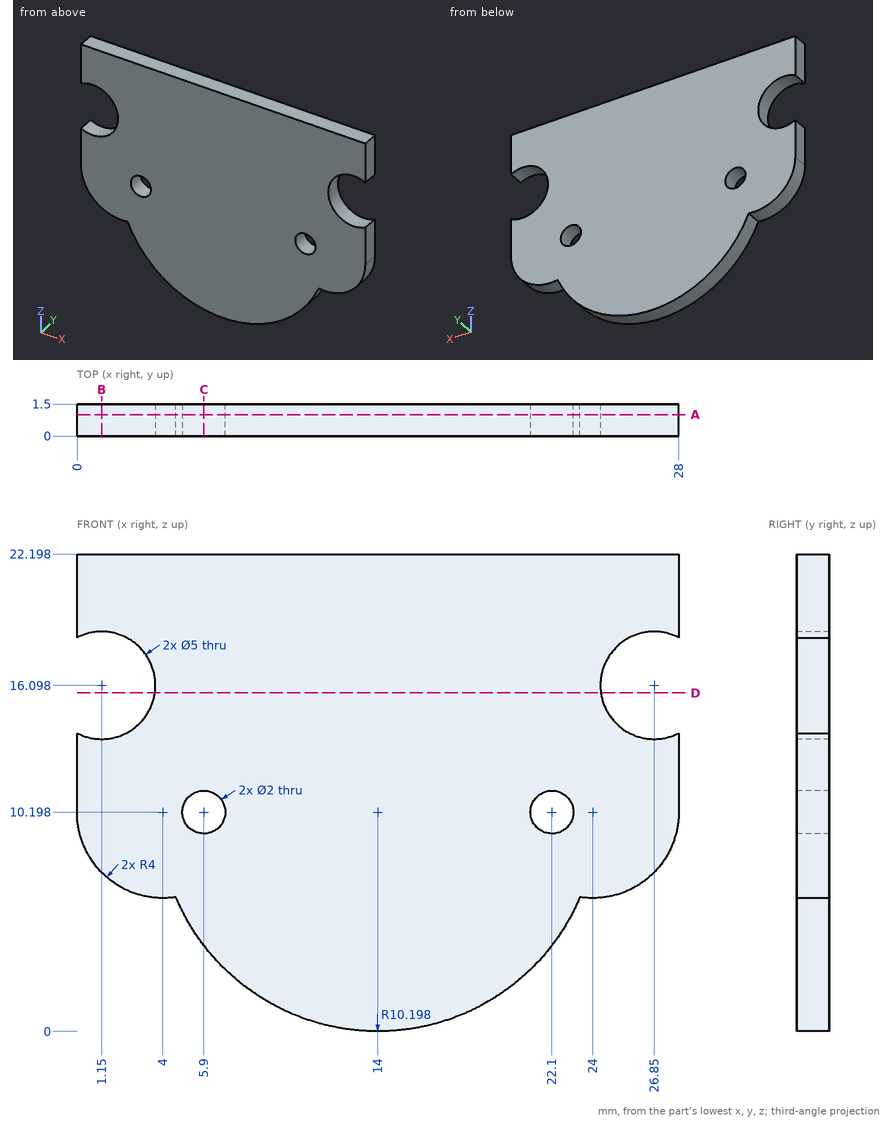
Design review of the part shown in the three views and the two pictorial views. Dimensions are in mm from the part's minimum x, y and z. Give positions to 0.01 mm unless a question says otherwise; leave off trailing zeros. Write each loop counter-clockwise with the first axis right and the second up, starting at its lowest first coordinate (ties: lowest second). Pieces come first, ordered by that corner, then holes. Notation, with made-up numbers: M 30,88 L 79,88 A28 ccw 79,121 Z; hole C -23.5,57 d5. An arc over 180 degrees is marked long. Return JSON: item names as keys, results as strings. Group by question number.
Item 1: Take a section at D-D (z = 15.75). Give the boundary of the cut face in (x, y), plus the area to 3 significant figures.
Item 2: Take a section at C-C (x = 5.9). Give the boundary of the cut face in (y, z), plus the area to 3 significant figures.
Item 3: Take a section at B-B (x = 1.15). Give the boundary of the cut face in (y, z), plus the area to 3 significant figures.
Item 4: Wall thickness on line 1 along X through (y, z) = (1.15, 10.25); line 2 along Z through (x, y) = (21.25, 0.5) (1 decimal); line 3 along Z through (x, y) = (1.15, 0.3): over which ranges is each line inside the solid? List them lowest first.
Item 5: Take a section at A-A (y = 1). Give the boundary of the cut face in (x, z), plus the area to 3 significant figures.
Return value:
{
 "1": {"outline": "M 3.63,0 L 24.37,0 L 24.37,1.5 L 3.63,1.5 Z", "area": "31.1 mm2"},
 "2": {"outline": "M 0,4 L 1.5,4 L 1.5,9.2 L 0,9.2 Z; M 0,11.2 L 1.5,11.2 L 1.5,22.2 L 0,22.2 Z", "area": "24.3 mm2"},
 "3": {"outline": "M 0,7.39 L 1.5,7.39 L 1.5,13.6 L 0,13.6 Z; M 0,18.6 L 1.5,18.6 L 1.5,22.2 L 0,22.2 Z", "area": "14.7 mm2"},
 "4": {"line 1": "x = 0 to 4.9, 6.9 to 21.1, 23.1 to 28", "line 2": "z = 3 to 9.7, 10.7 to 22.2", "line 3": "z = 7.39 to 13.6, 18.6 to 22.2"},
 "5": {"outline": "M 0,10.2 A4 ccw 4.6,6.24 A10.2 ccw 23.4,6.24 A4 ccw 28,10.2 L 28,13.88 A2.5 cw long 28,18.32 L 28,22.2 L 0,22.2 L 0,18.32 A2.5 cw long 0,13.88 Z; hole C 5.9,10.2 d2; hole C 22.1,10.2 d2", "area": "488 mm2"}
}
